Job drawing, mm, ordinate dimensions from the low corner. One solid piece. Give positions to 0.01 mm unless a question says otherwise; leave off trailing zeros. Order: outer loops, then holes, each group sorted by start corner. A loop starts at its lowest first (then second) coordinate and runs counter-clockwise, first axis right, second up.
1. Probe line 1 (Y direction, x = 250, z = 3.75); line 2 (X direction, y = 38, z = 1.3); line 3 (Y direction, x = 247.5, z = 1.55). List the from-to ranges inside material, lowest first.
2. Drop a flat-ended pin along its axis: pin 1 Ø15 at (x, y) = (30, 32.5) entering from -Z. Give the stop position or say it passes through.
3. Slice it at B-B on y = 32.5. List the corners of the cut face in (x, z).
4. Slice it at A-A on x = 250. List the corners of the cut face in (y, z).
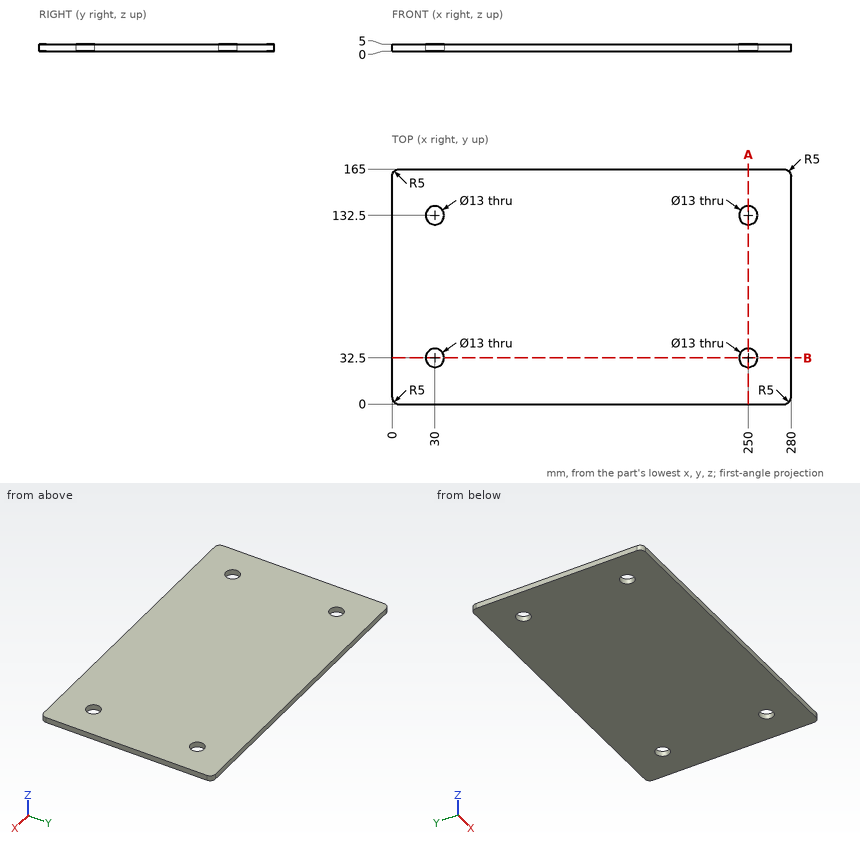
Data:
1. line 1: y = 0 to 26, 39 to 126, 139 to 165
1. line 2: x = 0 to 26.54, 33.46 to 246.54, 253.46 to 280
1. line 3: y = 0 to 26.5, 38.5 to 126.5, 138.5 to 165
2. pin 1: stops at z = 0
3. outline: (0, 0) - (23.5, 0) - (23.5, 5) - (0, 5) - close; (36.5, 0) - (243.5, 0) - (243.5, 5) - (36.5, 5) - close; (256.5, 0) - (280, 0) - (280, 5) - (256.5, 5) - close
4. outline: (0, 0) - (26, 0) - (26, 5) - (0, 5) - close; (39, 0) - (126, 0) - (126, 5) - (39, 5) - close; (139, 0) - (165, 0) - (165, 5) - (139, 5) - close
